from build123d import *

# Parameters (mm, degrees)
SKETCH3_W           = 50.8
SKETCH3_H           = 114.3
BOSS_EXTRUDE5_DEPTH = 50.8
DRAFT2_ANGLE        = 7
CHAMFER22_SIZE      = 35.56
CHAMFER22_SIZE_2    = 36.100146123
CHAMFER26_SIZE      = 12.7
CHAMFER26_SIZE_2    = 10.982965741
CHAMFER27_SIZE      = 27.462526176
CHAMFER27_SIZE_2    = 20.32
CHAMFER28_SIZE      = 32.227786218
CHAMFER28_SIZE_2    = 20.32
FILLET36_R          = 2.54
FILLET41_R          = 10.16
SHELL2_T            = -1.27


with BuildPart() as part:
    # Sketch3 → Boss-Extrude5 (new body)
    with BuildSketch(Plane.XY):
        Rectangle(SKETCH3_W, SKETCH3_H)
    extrude(amount=BOSS_EXTRUDE5_DEPTH)

    # Draft2
    draft2_faces = [part.faces().sort_by_distance(p)[0] for p in [
        (0, 0, 50.8),
        (25.4, 0, 25.4),
        (0, 0, 0),
        (-25.4, 0, 25.4),
    ]]
    draft(draft2_faces, Plane(origin=(-25.4, -57.15, 50.8), x_dir=(0, 0, -1), z_dir=(0, -1, 0)), DRAFT2_ANGLE)

    # Chamfer22
    # the kernel refuses this chamfer: 36.100146123, 35.56 mm, written as the material it takes off along each edge
    with BuildSketch(Plane(origin=(14.164548215, -148.655411614, 39.564548215), x_dir=(0.04243090311992196, 0.11662547522410431, -0.9922691756721962), z_dir=(0.1209742911513545, 0.9852565360152932, 0.1209742911513545)), Plane(origin=(-50.669727097, 148.655411614, 76.069727097), x_dir=(-0.04243090311992182, 0.11662547522410434, -0.9922691756721962), z_dir=(0.1209742911513545, -0.9852565360152932, -0.1209742911513545))) as chamfer22_piece_1:
        Polygon((CHAMFER22_SIZE * 0.999610675702, CHAMFER22_SIZE * 0.0279015595125), (-CHAMFER22_SIZE_2 * 0.0427448365612, CHAMFER22_SIZE_2 * 0.999086021807), (0, 0), align=None)
    extrude(amount=301.759808092, mode=Mode.SUBTRACT)
    with BuildSketch(Plane(origin=(14.164548215, -148.655411614, 11.235451785), x_dir=(0.04160965436003197, 0.11672908614577471, 0.9922917701521116), z_dir=(0.1209742911513545, 0.9852565360152932, -0.1209742911513545)), Plane(origin=(-50.669727097, 148.655411614, -25.269727097), x_dir=(-0.04160965436003206, 0.11672908614577471, 0.9922917701521116), z_dir=(0.1209742911513545, -0.9852565360152932, 0.1209742911513545))) as chamfer22_piece_2:
        Polygon((CHAMFER22_SIZE_2 * 0.999633437363, -CHAMFER22_SIZE_2 * 0.0270738052216), (-CHAMFER22_SIZE * 0.0419175116292, -CHAMFER22_SIZE * 0.999121074855), (0, 0), align=None)
    extrude(amount=301.759808092, mode=Mode.SUBTRACT)

    # Chamfer26
    # the kernel refuses this chamfer: 12.7, 10.982965741 mm, written as the material it takes off along each edge
    with BuildSketch(Plane(origin=(62.353919786, 57.15, 45.600752144), x_dir=(-0.10253351623411874, -0.9895888066791988, 0.10099936506685082), z_dir=(-0.7017569520656596, 0, -0.7124164373647731))) as chamfer26_piece_1:
        Polygon((CHAMFER26_SIZE * 0.999621916911, CHAMFER26_SIZE * 0.0274958766106), (CHAMFER26_SIZE_2 * 0.14392356894, CHAMFER26_SIZE_2 * 0.989588806705), (0, 0), align=None)
    extrude(amount=116.368475455, mode=Mode.SUBTRACT)
    with BuildSketch(Plane(origin=(20.200752144, 57.15, 87.753919786), x_dir=(0.10099936506686123, -0.9895888066791988, -0.10253351623410831), z_dir=(-0.7124164373647012, 0, -0.7017569520657325))) as chamfer26_piece_2:
        Polygon((CHAMFER26_SIZE * 0.999621916911, -CHAMFER26_SIZE * 0.0274958766106), (CHAMFER26_SIZE_2 * 0.14392356894, -CHAMFER26_SIZE_2 * 0.989588806705), (0, 0), align=None)
    extrude(amount=116.368475455, mode=Mode.SUBTRACT)

    # Chamfer27
    # the kernel refuses this chamfer: 27.462526176, 20.32 mm, written as the material it takes off along each edge
    with BuildSketch(Plane(origin=(85.378052857, 57.15, -16.24516911), x_dir=(-0.10283002660704509, -0.9892058931774511, -0.10439198499403901), z_dir=(-0.7124164373647012, 0, 0.7017569520657325))) as chamfer27_piece_1:
        Polygon((CHAMFER27_SIZE * 0.999690938869, -CHAMFER27_SIZE * 0.0248601439751), (CHAMFER27_SIZE_2 * 0.146532252091, -CHAMFER27_SIZE_2 * 0.989205893177), (0, 0), align=None)
    extrude(amount=179.645229373, mode=Mode.SUBTRACT)

    # Chamfer28
    # the kernel refuses this chamfer: 32.227786218, 20.32 mm, written as the material it takes off along each edge
    with BuildSketch(Plane(origin=(50.702210768, 57.15, -69.17266836), x_dir=(0.10631921382033309, -0.9888013870052722, 0.10472841939548341), z_dir=(-0.7017569520656596, 0, 0.7124164373647731))) as chamfer28_piece_1:
        Polygon((CHAMFER28_SIZE * 0.999755198418, CHAMFER28_SIZE * 0.0221256235269), (CHAMFER28_SIZE_2 * 0.149237451923, CHAMFER28_SIZE_2 * 0.988801387005), (0, 0), align=None)
    extrude(amount=205.453325716, mode=Mode.SUBTRACT)

    # Fillet36
    fillet36_edges = [part.edges().sort_by_distance(p)[0] for p in [
        (13.620964483, 57.15, 11.778226285),
        (7.018121545, 57.15, 32.419663344),
        (-13.620970138, 57.15, 39.021756036),
        (-7.0181272, 57.15, 18.380318978),
    ]]
    fillet(fillet36_edges, radius=FILLET36_R)

    # Fillet41
    fillet41_edges = [part.edges().sort_by_distance(p)[0] for p in [
        (0, -13.528827954, 50.628730432),
        (0, -15.876331706, 0.368905118),
        (25.400607617, -13.597419467, 25.591459835),
        (-24.841008934, -15.876331706, 25.587241799),
    ]]
    fillet(fillet41_edges, radius=FILLET41_R)

    # Shell2
    shell2_openings = [part.faces().sort_by_distance(p)[0] for p in [
        (0, -57.15, 25.396792281),
    ]]
    offset(amount=SHELL2_T, openings=shell2_openings)


solid = part.part
Work out the finished part from the listing and answer in its coordinate system (mm). A direction names the side the tool comes from. Coordinates: 2 decimals unless noted, no trailing zeros. Write each loop counter-clockwise with the first axis right and the second up, starting at its lowest first coordinate (ties: lowest second). Pieces come first, ordered by that corner, then holes. Notation, with made-up numbers: M 47,-21 L 78,-21 A23 ccw 78,18 Z; hole C 1,16 d2. An arc over 180 degrees is marked long. Answer as CSV lines item,"result". Start each with the question number.
Item 1: A tool of negligible diameter and unlimited length cuts with its end or side. For faces 5 (the face through (-15.588, 49.762, 42.206)), 6 (the face through (-0.11, -8.33, 47.88)), from which of +Z, -Z, +X, -X, +Y, -Y can it reach the whole face along a straight path? Write none if from no direction.
Item 2: Section A-A on y = 48 is taken. Write down the section's boundary in (x, z), and give its area (3 significant figures).
Item 3: Consider L1, parallel to X at y = 36.5, z = 0; L2, parallel to Z at x = -15.5, y = 26; L3, parallel to X at y = 49, z = 25.5. Determine where each line is inside the solid, lowest interval first.
Item 4: Flat-ended cylindrical pins translate along their axes: P1, Ø3, axis at x = 0.5, z = 47, coming from the +Y side; P2, Ø5, axis at y = 30, z = 16.5, coming from the -X side; P3, Ø1, axis at y = -5.5, z = 20, coming from the -X side. Find the tip coordinate at first contact, or state that the pin passes through.
Item 5: Determine the mould class of faces 1 (the face through (-12.89, -6.22, 12.9)), 2 (the face through (6.7, 56.8, 32.48)), 3 (the face through (-7.022, 56.763, 18.77)), 4 (the face through (-6.536, 55.686, 19.237)) for opening direction Z: released by +Z, released by -Z, zero draft, split by the parting line, or undercut.
Checks:
1,face 5,"none"
1,face 6,"+Z, -Y"
2,outline,"M -28.15,33.75 L 8.08,-3.03 L 28.99,18.2 L -7.48,54.12 Z; hole M -26.06,33.63 L 7.97,-0.92 L 26.85,18.24 L -7.42,52 Z"
2,area,"230 mm²"
3,L1,"x = -2.43 to -0.46, 10.59 to 12.4"
3,L2,"z = 6.29 to 8.29, 43.19 to 45"
3,L3,"x = -19.37 to -17.4, 18.66 to 20.75"
4,P1,"stops at y = 49.68"
4,P2,"stops at x = -25.89"
4,P3,"stops at x = -21.94"
5,face 1,"undercut"
5,face 2,"released by +Z"
5,face 3,"released by -Z"
5,face 4,"undercut"
